Geometry check sheet. Reference: the model listing, model coordinates, mm. Face numbers are marked on the shaded views. A direction names the side the tool comes from. Round coordinates to 2 decimals unless told otherwise and drop trailing zeros. Order: outer loops, then holes, each group sorted by start corner. A loop starts at its lowest first (then second) coordinate and runs counter-clockwise, first axis right, second up.
(1) Release check for a two-part mould opening along X. For the marked faces 1, 2, 3 and 4 record: +X half, -X half, draft (parallel to the pull), parting line (faces both ways), or undercut.
(2) Go/stop test with flat-tipped pins: pin 1 (5 mm diameter, centred on x = 126.5, y = 32, fed in from -Z); pin 2 (2 mm diameter, centred on x = 61, y = 50.5, fed in from +Z). Record where each tip stops, or that it passes through.
(3) Set-up check for the marked faces 5 and 6: record each of +Z, -Z, +X, -X, +Y, -Y from which the full face is reachable in a straight line by a thin tool's end or side.
(4) Sectioned sample at B-B (y = 79.5). Record the boundary of the cut face in (x, z), plus the area to 3 significant figures.
(5) Sectioned sample at C-C (x = 120). Record the boundary of the cut face in (y, z), plus the area to 3 significant figures.
(6) Sectioned sample at D-D (z = 20). Record the boundary of the cut face in (x, y).
(7) Sectioned sample at A-A (z = 13). Record the boundary of the cut face in (x, y), plus the area to 3 significant figures.
(8) Material ranges on line 1 along Y through (x, z) = (49, 35); line 2 along X through (y, z) = (54, 6); line 3 along Z through (x, y) = (70.5, 28), recorded low to high.
from build123d import *

# Parameters (mm, degrees)
SKETCH_W        = 134
SKETCH_H        = 90
PAD_DEPTH       = 38
SKETCH001_W     = 130
SKETCH001_H     = 86
POCKET_DEPTH    = 36
SKETCH003_R     = 4
POCKET001_DEPTH = 5
SKETCH004_R     = 4
POCKET002_DEPTH = 5


with BuildPart() as part:
    # Sketch → Pad (new body)
    with BuildSketch(Plane.XY):
        with Locations((77, 55)):
            Rectangle(SKETCH_W, SKETCH_H)
    extrude(amount=PAD_DEPTH)

    # Sketch001 (on Face6 of Pad) → Pocket (cut)
    with BuildSketch(Plane.XY.offset(38)):
        with Locations((77, 55)):
            Rectangle(SKETCH001_W, SKETCH001_H)
    extrude(amount=-POCKET_DEPTH, mode=Mode.SUBTRACT)

    # Sketch003 (on Face1 of Pocket) → Pocket001 (cut)
    with BuildSketch(Plane.XZ.offset(-10)):
        with Locations((119.765617, 19.578506)):
            Circle(SKETCH003_R)
    extrude(amount=-POCKET001_DEPTH, mode=Mode.SUBTRACT)

    # Sketch004 (on Face1 of Pad) → Pocket002 (cut)
    with BuildSketch(Plane.XZ.offset(-10)):
        with Locations((120, 20)):
            Circle(SKETCH004_R)
    extrude(amount=-POCKET002_DEPTH, mode=Mode.SUBTRACT)


solid = part.part
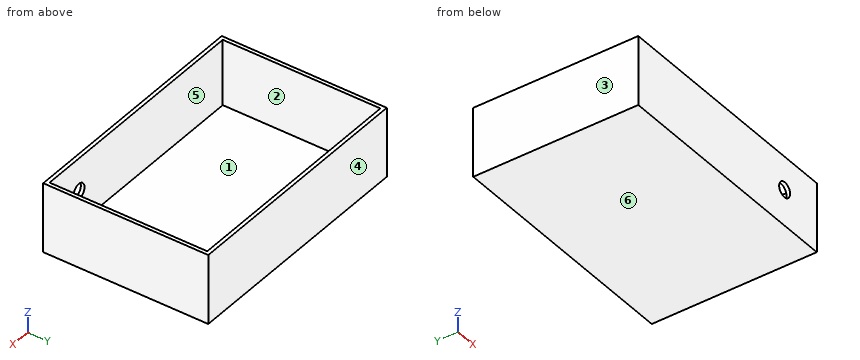
Answer below:
1. face 1: undercut
1. face 2: undercut
1. face 3: -X half
1. face 4: draft
2. pin 1: stops at z = 0
2. pin 2: stops at z = 2
3. face 5: +Z
3. face 6: -Z, +X, -X, +Y, -Y
4. outline: (10, 0) - (144, 0) - (144, 38) - (142, 38) - (142, 2) - (12, 2) - (12, 38) - (10, 38) - close
4. area: 412 mm2
5. outline: (10, 0) - (100, 0) - (100, 38) - (98, 38) - (98, 2) - (12, 2) - (12, 15.59) - (10, 15.59) - close; (10, 24) - (12, 24) - (12, 38) - (10, 38) - close
5. area: 307 mm2
6. outline: (10, 10) - (115.79, 10) - (115.79, 12) - (12, 12) - (12, 98) - (142, 98) - (142, 12) - (124, 12) - (124, 10) - (144, 10) - (144, 100) - (10, 100) - close
7. outline: (10, 10) - (144, 10) - (144, 100) - (10, 100) - close; hole (12, 12) - (142, 12) - (142, 98) - (12, 98) - close
7. area: 880 mm2
8. line 1: y = 10 to 12, 98 to 100
8. line 2: x = 10 to 12, 142 to 144
8. line 3: z = 0 to 2
